from build123d import *

# Parameters (mm, degrees)
BOSS_EXTRUDE1_DEPTH = 5
SKETCH2_OUTSIDE_W   = 24.604
SKETCH2_OUTSIDE_H   = 26.078
SKETCH2_OUTSIDE_R   = 4.763139721
CUT_EXTRUDE2_DEPTH  = 5
CUT_EXTRUDE2_TAPER  = 45
SKETCH5_R           = 6.5
BOSS_EXTRUDE2_DEPTH = 1
SKETCH6_R           = 2.5
BOSS_EXTRUDE3_DEPTH = 25


with BuildPart() as part:
    # Sketch1 → Boss-Extrude1 (new body)
    with BuildSketch(Plane.XY):
        Polygon((0, -5.5), (4.763139721, -2.75), (4.763139721, 2.75), (0, 5.5), (-4.763139721, 2.75), (-4.763139721, -2.75), align=None)
    extrude(amount=-BOSS_EXTRUDE1_DEPTH)

    # Sketch2 outside → Cut-Extrude2 (cut)
    with BuildSketch(Plane.XY):
        Rectangle(SKETCH2_OUTSIDE_W, SKETCH2_OUTSIDE_H)
        Circle(SKETCH2_OUTSIDE_R, mode=Mode.SUBTRACT)
    extrude(amount=-CUT_EXTRUDE2_DEPTH, taper=CUT_EXTRUDE2_TAPER, mode=Mode.SUBTRACT)

    # Sketch5 → Boss-Extrude2 (add)
    with BuildSketch(Plane(origin=(0, 0, -5), x_dir=(-1, 0, 0), z_dir=(0, 0, -1))):
        Circle(SKETCH5_R)
    extrude(amount=BOSS_EXTRUDE2_DEPTH)

    # Sketch6 → Boss-Extrude3 (add)
    with BuildSketch(Plane(origin=(0, 0, -6), x_dir=(-1, 0, 0), z_dir=(0, 0, -1))):
        Circle(SKETCH6_R)
    extrude(amount=BOSS_EXTRUDE3_DEPTH)


solid = part.part
Geometry check sheet. Reference: the model listing, model coordinates, mm. A direction names the side the tool comes from. Give positions to 0.01 mm unless a question says otherwise; leave off trailing zeros. Order: outer loops, then holes, each group sorted by start corner. A loop starts at its lowest first (then second) coordinate and runs counter-clockwise, first axis right, second up. Notation, with made-up numbers: (8.5, 50) - (29.5, 50) arc R5 ccw to (29.5, 59) - close; hole circle Ø1 at (-38, 67.5). An arc over 180 degrees is marked (long way). Answer as a JSON object with one key per item and string values.
(1) Tool access check on faces 1 (the flat face through (2.41, 4.11, -2.46)), 2 (the flat face through (-2.348, 4.144, -2.465)), 3 (the flat face through (-4.763, 0, -2)). Record the directions out of +Z, -Z, +X, -X, +Y, -Y that give a thin tool (end or side, any length) a straight path to the whole face; none if there is none.
Report:
{"face 1": "+Z, +X, +Y", "face 2": "+Z, -X, +Y", "face 3": "+Z, -X, +Y, -Y"}
(2) Depth check by flat-ended pin: pin 1 Ø1.5 at (y, z) = (-1.5, -3) entering from -X; pin 2 Ø6.5 at (x, y) = (1.5, 0.5) entering from +Z; pin 3 Ø1 at (x, y) = (3.5, 4.5) entering from +Z; pin 4 Ø1 at (y, z) = (1.5, -12) entering from -X. Enter the tip coordinate at first touch or a pass-through.
Report:
{"pin 1": "x = -4.76", "pin 2": "z = 0", "pin 3": "z = -5", "pin 4": "x = -2.29"}
(3) Cross-section at A-A (z = -22.5). Record the cut outline in (x, y).
Report:
{"outline": "circle Ø5 at (0, 0)"}
(4) Material ranges on line 1 (Z direction, x = 4, y = -0.5); line 2 (Z direction, x = 2.25, y = 4.25); line 3 (X direction, y = -0.75, z = -13), recorded low to high.
Report:
{"line 1": "-6 to 0", "line 2": "-6 to -5", "line 3": "-2.38 to 2.38"}
